```python
from build123d import *

# Parameters (mm, degrees)
SKETCH1_R               = 215
SKETCH1_R_2             = 175
RING_DEPTH              = 12
SKETCH2_R               = 40
HUB_DEPTH               = 40
SKETCH3_W               = 20
SKETCH3_H               = 137
SPOKES_DEPTH            = 12
SKETCH4_R               = 6
BORE_DEPTH              = 40
SKETCH5_R               = 11
BEARING_SEAT_LOW_DEPTH  = 7
SKETCH6_R               = 11
BEARING_SEAT_HIGH_DEPTH = 7
SKETCH7_R               = 216
SKETCH7_R_2             = 212
BAND_RABBET_DEPTH       = 3
SKETCH8_R               = 216
SKETCH8_R_2             = 212
COVER_RABBET_DEPTH      = 3
SKETCH9_R               = 2.75
ROD_HOLES_DEPTH         = 12
SKETCH10_R              = 1.25
GROMMET_SCREWS_DEPTH    = 8


with BuildPart() as part:
    # Sketch1 → Ring (new body)
    with BuildSketch(Plane.XY):
        Circle(SKETCH1_R)
        Circle(SKETCH1_R_2, mode=Mode.SUBTRACT)
    extrude(amount=RING_DEPTH)



with BuildPart() as body_2:
    # Sketch2 → Hub (new body)
    with BuildSketch(Plane.XY):
        Circle(SKETCH2_R)
    extrude(amount=HUB_DEPTH)


with BuildPart() as part_1:
    add(part.part)

    add(body_2.part)  # Spokes merges body 2
    # Sketch3 → Spokes (add)
    with BuildSketch(Plane.XY):
        Polygon((40.181374079, 2.541097618), (170.476116812, 44.876425847), (164.295776924, 63.897556173), (34.001034192, 21.562227944), align=None)
        with Locations((0, 107.5)):
            Rectangle(SKETCH3_W, SKETCH3_H)
        Polygon((-34.001034192, 21.562227944), (-164.295776924, 63.897556173), (-170.476116812, 44.876425847), (-40.181374079, 2.541097618), align=None)
        Polygon((-31.013794783, -25.673810258), (-111.540374347, -136.509138487), (-95.36003446, -148.264843533), (-14.833454896, -37.429515304), align=None)
        Polygon((14.833454896, -37.429515304), (95.36003446, -148.264843533), (111.540374347, -136.509138487), (31.013794783, -25.673810258), align=None)
    extrude(amount=SPOKES_DEPTH)

    # Sketch4 → Bore (cut)
    with BuildSketch(Plane.XY):
        Circle(SKETCH4_R)
    extrude(amount=BORE_DEPTH, mode=Mode.SUBTRACT)

    # Sketch5 → Bearing_seat_low (cut)
    with BuildSketch(Plane.XY):
        Circle(SKETCH5_R)
    extrude(amount=BEARING_SEAT_LOW_DEPTH, mode=Mode.SUBTRACT)

    # Sketch6 → Bearing_seat_high (cut)
    with BuildSketch(Plane.XY.offset(33)):
        Circle(SKETCH6_R)
    extrude(amount=BEARING_SEAT_HIGH_DEPTH, mode=Mode.SUBTRACT)

    # Sketch7 → Band_rabbet (cut)
    with BuildSketch(Plane.XY):
        Circle(SKETCH7_R)
        Circle(SKETCH7_R_2, mode=Mode.SUBTRACT)
    extrude(amount=BAND_RABBET_DEPTH, mode=Mode.SUBTRACT)

    # Sketch8 → Cover_rabbet (cut)
    with BuildSketch(Plane.XY.offset(9)):
        Circle(SKETCH8_R)
        Circle(SKETCH8_R_2, mode=Mode.SUBTRACT)
    extrude(amount=COVER_RABBET_DEPTH, mode=Mode.SUBTRACT)

    # Sketch9 → Rod_holes (cut)
    with BuildSketch(Plane.XY):
        with Locations((198.770811906, 64.584551824)):
            Circle(SKETCH9_R)
        with Locations((0, 209)):
            Circle(SKETCH9_R)
        with Locations((-198.770811906, 64.584551824)):
            Circle(SKETCH9_R)
        with Locations((-122.847117729, -169.084551824)):
            Circle(SKETCH9_R)
        with Locations((122.847117729, -169.084551824)):
            Circle(SKETCH9_R)
    extrude(amount=ROD_HOLES_DEPTH, mode=Mode.SUBTRACT)

    # Sketch10 → Grommet_screws (cut)
    with BuildSketch(Plane.XY.offset(32)):
        with Locations((21.213203436, 21.213203436)):
            Circle(SKETCH10_R)
        with Locations((-21.213203436, 21.213203436)):
            Circle(SKETCH10_R)
        with Locations((-21.213203436, -21.213203436)):
            Circle(SKETCH10_R)
        with Locations((21.213203436, -21.213203436)):
            Circle(SKETCH10_R)
    extrude(amount=GROMMET_SCREWS_DEPTH, mode=Mode.SUBTRACT)


solid = part_1.part
```
Model file for the job. Use its own axes, mm. A direction names the side the tool comes from. Coordinates: 2 decimals unless noted, no trailing zeros. Loops run counter-clockwise (first coordinate to the right, second up) from the corner with the lowest first, then second, coordinate; pieces in that order, holes last. Notation, with made-up numbers: (56.5, 30) - (104.5, 30) arc R25 ccw to (104.5, 52) - close; hole circle Ø9 at (32, 29.5). An arc over 180 degrees is marked (long way). Write item = value, one per line. Start each with the question number.
Item 1: Wall check: probe 1 along Y at (x, z) = (0, 4); probe 2 along Y at (x, z) = (0, 37); probe 3 along X at (y, z) = (0, 27). Give the ranges that are in metal, low to high. Write a range as [from, to].
Item 2: Pull direction Y, two halves, no side cores. Call faces 1 (the face through (113.97, 178.76, 10.48)), 2 (the face through (-101.727, 142.396, 5.916)), 3 (the face through (-1, -15, 0)): +Y half, -Y half, draft (parallel to the pull), parting line (faces both ways), or undercut.
Item 3: Drop flat-ended pins along their axis: pin 1 Ø6.5 at (x, y) = (-5, -3.5) entering from +Z; pin 2 Ø4 at (y, z) = (31, 29) entering from -X; pin 3 Ø20 at (x, y) = (0, 0) entering from -Z; pin 4 Ø4 at (x, y) = (21.21, -21.21) entering from -Z. Give the stop position or say it passes through.
Item 4: 3-axis set-ups, long thin cutter, end or side, ignore diameter. For faces 4 (the face through (-2.38, -10.74, 3.45)), 5 (the face through (-2.38, -10.74, 36.45)), 6 (the face through (103.814, 23.217, 5.916)), 7 (the face through (8, -8, 40)): which of +Z, -Z, +X, -X, +Y, -Y reach the whole face in a straight line?
Item 5: Saw through at A-A, the plane y = -76. List the corners of the cut face in (x, z), then the cut area to 3 significant figures.
Item 6: Saw through at C-C, the plane z = 26.5. List the corners of the cut face in (x, y).
Item 7: Saw through at B-B, the plane x = 72. List the corners of the cut face in (y, z), then the cut area to 3 significant figures.
Answers:
q1.probe_1 = [-215, -175], [-40, -11], [11, 206.25], [211.75, 215]
q1.probe_2 = [-40, -11], [11, 40]
q1.probe_3 = [-40, -6], [6, 40]
q2.face_1 = parting line
q2.face_2 = undercut
q2.face_3 = draft
q3.pin_1 = 33
q3.pin_2 = -27.55
q3.pin_3 = 7
q3.pin_4 = 0
q4.face_4 = -Z
q4.face_5 = +Z
q4.face_6 = +Z, -Z
q4.face_7 = +Z, +X, -X, +Y, -Y
q5.outline = (-201.12, 3) - (-197.91, 3) - (-197.91, 0) - (-157.64, 0) - (-157.64, 12) - (-197.91, 12) - (-197.91, 9) - (-201.12, 9) - close; (-67.58, 0) - (-42.86, 0) - (-42.86, 12) - (-67.58, 12) - close; (42.86, 0) - (67.58, 0) - (67.58, 12) - (42.86, 12) - close; (157.64, 0) - (197.91, 0) - (197.91, 3) - (201.12, 3) - (201.12, 9) - (197.91, 9) - (197.91, 12) - (157.64, 12) - close
q5.area = 1,600 mm2
q6.outline = circle Ø80 at (0, 0); hole circle Ø12 at (0, 0)
q7.outline = (-202.59, 3) - (-199.4, 3) - (-199.4, 0) - (-159.5, 0) - (-159.5, 12) - (-199.4, 12) - (-199.4, 9) - (-202.59, 9) - close; (-116.11, 0) - (-82.09, 0) - (-82.09, 12) - (-116.11, 12) - close; (12.88, 0) - (33.91, 0) - (33.91, 12) - (12.88, 12) - close; (159.5, 0) - (199.4, 0) - (199.4, 3) - (202.59, 3) - (202.59, 9) - (199.4, 9) - (199.4, 12) - (159.5, 12) - close
q7.area = 1,660 mm2
